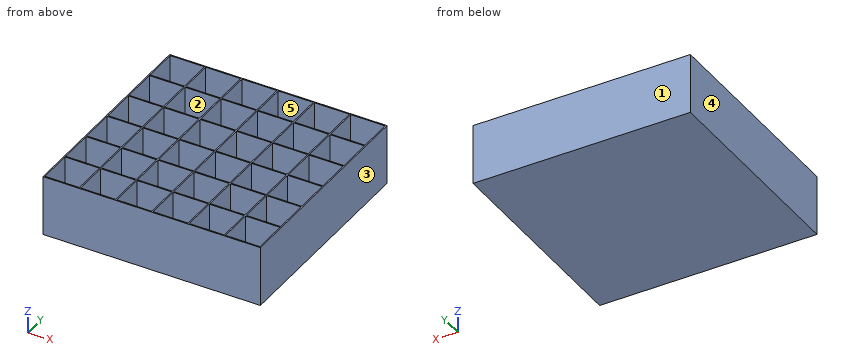
```python
from build123d import *

# Parameters (mm, degrees)
SKETCH_W      = 180
SKETCH_H      = 180
PAD_DEPTH     = 50
SKETCH001_W   = 28.499999
SKETCH001_H   = 28.499999
SKETCH001_W_2 = 28.5
SKETCH001_H_2 = 29.000001
SKETCH001_H_3 = 29
SKETCH001_W_3 = 29.000001
SKETCH001_H_4 = 28.5
SKETCH001_W_4 = 28.977006
SKETCH001_W_5 = 29
SKETCH001_W_6 = 28.975581
POCKET_DEPTH  = 49


with BuildPart() as part:
    # Sketch → Pad (new body)
    with BuildSketch(Plane.XY):
        Rectangle(SKETCH_W, SKETCH_H)
    extrude(amount=PAD_DEPTH)

    # Sketch001 (on Face6 of Pad) → Pocket (cut)
    with BuildSketch(Plane.XY.offset(50)):
        with Locations((-74.75, 74.75)):
            Rectangle(SKETCH001_W, SKETCH001_H)
        with Locations((-74.750001, 45)):
            Rectangle(SKETCH001_W_2, SKETCH001_H_2)
        with Locations((-74.750001, 15)):
            Rectangle(SKETCH001_W_2, SKETCH001_H_3)
        with Locations((-45, 74.750001)):
            Rectangle(SKETCH001_W_3, SKETCH001_H_4)
        with Locations((-45.011498, 45)):
            Rectangle(SKETCH001_W_4, SKETCH001_H_2)
        with Locations((-45, 15)):
            Rectangle(SKETCH001_W_3, SKETCH001_H_3)
        with Locations((-15, 74.750001)):
            Rectangle(SKETCH001_W_5, SKETCH001_H_4)
        with Locations((-15, 45)):
            Rectangle(SKETCH001_W_5, SKETCH001_H_2)
        with Locations((-15, 15)):
            Rectangle(SKETCH001_W_5, SKETCH001_H_3)
        with Locations((15, 74.750001)):
            Rectangle(SKETCH001_W_5, SKETCH001_H_4)
        with Locations((15, 45)):
            Rectangle(SKETCH001_W_5, SKETCH001_H_2)
        with Locations((15.01221, 15)):
            Rectangle(SKETCH001_W_6, SKETCH001_H_3)
        with Locations((15, -15)):
            Rectangle(SKETCH001_W_5, SKETCH001_H_3)
        with Locations((15, -45)):
            Rectangle(SKETCH001_W_5, SKETCH001_H_2)
        with Locations((15, -74.750001)):
            Rectangle(SKETCH001_W_5, SKETCH001_H_4)
        with Locations((-74.750001, -15)):
            Rectangle(SKETCH001_W_2, SKETCH001_H_3)
        with Locations((-45, -15)):
            Rectangle(SKETCH001_W_3, SKETCH001_H_3)
        with Locations((-15, -15)):
            Rectangle(SKETCH001_W_5, SKETCH001_H_3)
        with Locations((-15, -45)):
            Rectangle(SKETCH001_W_5, SKETCH001_H_2)
        with Locations((-15, -74.750001)):
            Rectangle(SKETCH001_W_5, SKETCH001_H_4)
        with Locations((-74.750001, -45)):
            Rectangle(SKETCH001_W_2, SKETCH001_H_2)
        with Locations((-45, -45)):
            Rectangle(SKETCH001_W_3, SKETCH001_H_2)
        with Locations((-45, -74.750001)):
            Rectangle(SKETCH001_W_3, SKETCH001_H_4)
        with Locations((-74.750001, -74.750001)):
            Rectangle(SKETCH001_W_2, SKETCH001_H_4)
        with Locations((45, 74.750001)):
            Rectangle(SKETCH001_W_3, SKETCH001_H_4)
        with Locations((45, 45)):
            Rectangle(SKETCH001_W_3, SKETCH001_H_2)
        with Locations((45, 15)):
            Rectangle(SKETCH001_W_3, SKETCH001_H_3)
        with Locations((45, -15)):
            Rectangle(SKETCH001_W_3, SKETCH001_H_3)
        with Locations((45, -45)):
            Rectangle(SKETCH001_W_3, SKETCH001_H_2)
        with Locations((45, -74.750001)):
            Rectangle(SKETCH001_W_3, SKETCH001_H_4)
        with Locations((74.750001, 74.750001)):
            Rectangle(SKETCH001_W_2, SKETCH001_H_4)
        with Locations((74.750001, 45)):
            Rectangle(SKETCH001_W_2, SKETCH001_H_2)
        with Locations((74.750001, 15)):
            Rectangle(SKETCH001_W_2, SKETCH001_H_3)
        with Locations((74.750001, -15)):
            Rectangle(SKETCH001_W_2, SKETCH001_H_3)
        with Locations((74.750001, -45)):
            Rectangle(SKETCH001_W_2, SKETCH001_H_2)
        with Locations((74.750001, -74.750001)):
            Rectangle(SKETCH001_W_2, SKETCH001_H_4)
    extrude(amount=-POCKET_DEPTH, mode=Mode.SUBTRACT)


solid = part.part
```
The model under review builds one solid part; all positions refer to its coordinate system, in mm. Face numbers are marked on the shaded views. A direction names the side the tool comes from. Give positions to 0.01 mm unless a question says otherwise; leave off trailing zeros. Write each loop counter-clockwise with the first axis right and the second up, starting at its lowest first coordinate (ties: lowest second). Pieces come first, ordered by that corner, then holes.
(1) To check wall thickness, follow L1, parallel to Z at x = -50.5, y = -44. State the ranges of the line that lie inside material, in increasing order.
(2) Tool access review of the marked faces 4 and 5: name each direction out of +Z, -Z, +X, -X, +Y, -Y from which nothing blocks a thin tool from reaching the whole face with its end or side.
(3) Consider section A-A, the plane y = -40.5. Give the boundary of the cut face in (x, z).
(4) Consider section C-C, the plane z = 9. Give the number of separate pieces and of enclosed holes in the cut face, and give its area (3 significant figures).
(5) The part is to be moulded in two halves that separate along Y. For the marked faces 1, 2 and 3, say which applies: released by +Y, released by -Y, zero draft, split by the parting line, or undercut.
(6) For P1, Ø12, axis at x = -43.5, y = 67.5, coming from the +Z side, flat-tipped, find the tip position at first contact; note if it passes through.
Returned:
1. L1: z = 0 to 1
2. face 4: +Z, -Z, -X, +Y, -Y
2. face 5: +Z
3. outline: (-90, 0) - (90, 0) - (90, 50) - (89, 50) - (89, 1) - (60.5, 1) - (60.5, 50) - (59.5, 50) - (59.5, 1) - (30.5, 1) - (30.5, 50) - (29.5, 50) - (29.5, 1) - (0.5, 1) - (0.5, 50) - (-0.5, 50) - (-0.5, 1) - (-29.5, 1) - (-29.5, 50) - (-30.5, 50) - (-30.5, 1) - (-59.5, 1) - (-59.5, 50) - (-60.5, 50) - (-60.5, 1) - (-89, 1) - (-89, 50) - (-90, 50) - close
4. separate pieces: 1
4. enclosed holes: 36
4. area: 2,470 mm2
5. face 1: released by +Y
5. face 2: undercut
5. face 3: zero draft
6. P1: stops at z = 1
